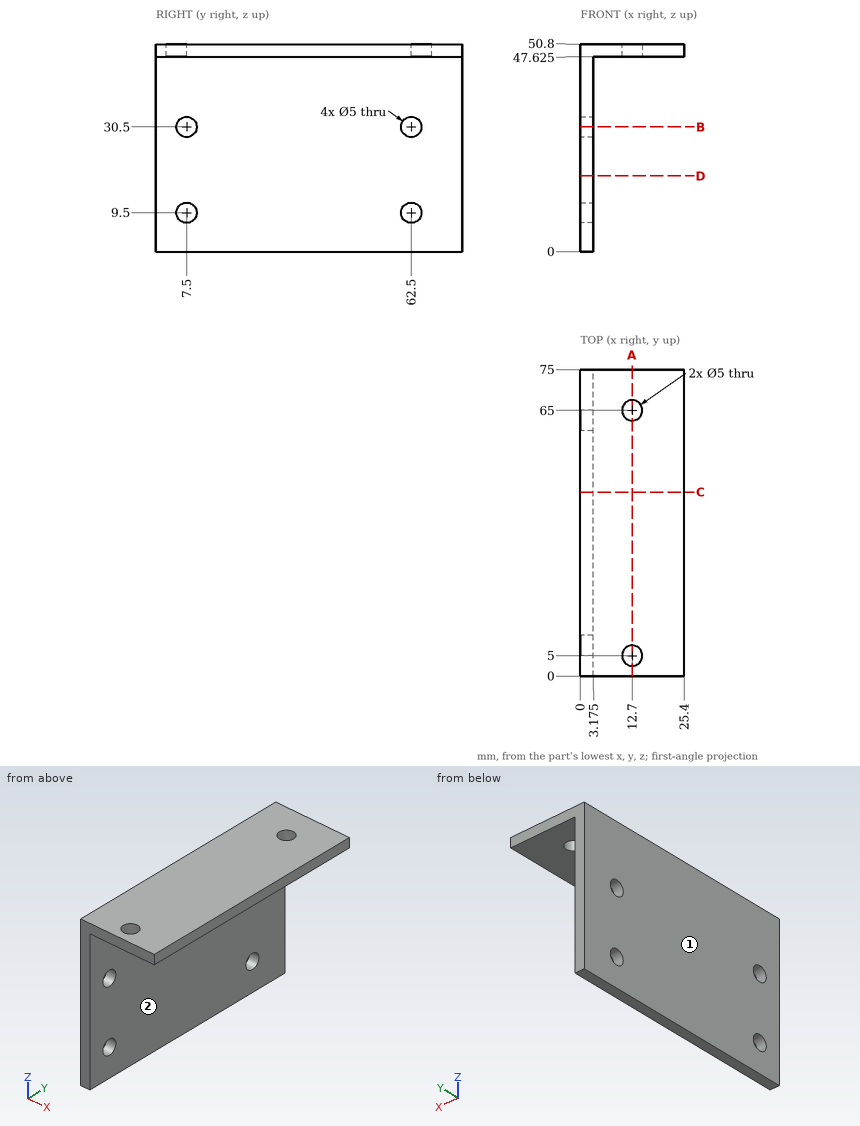
Can you work these out from the drawing? Everything is in mm from the part's minimum corner. A direction names the side the tool comes from. Round coordinates to 2 decimals unless told otherwise and drop trailing zeros. Write each loop counter-clockwise with the first axis right and the second up, starting at its lowest first coordinate (ties: lowest second). Pieces come first, ordered by that corner, then holes. Notation, with made-up numbers: (75, -27.5) - (124, -27.5) arc R27 ccw to (124, -0.5) - close; hole circle Ø11 at (50, 48.25). An arc over 180 degrees is marked (long way). Use a Markdown table: item, result.
Q1. I want a section at A-A (x = 12.7). List the corners of the cut face in (y, z) for me (3 decimals), plus the area to 3 significant figures.
Output values:
| item | result |
|---|---|
| outline | (0, 47.625) - (2.5, 47.625) - (2.5, 50.8) - (0, 50.8) - close; (7.5, 47.625) - (62.5, 47.625) - (62.5, 50.8) - (7.5, 50.8) - close; (67.5, 47.625) - (75, 47.625) - (75, 50.8) - (67.5, 50.8) - close |
| area | 206 mm2 |
Q2. For pin 1 (6.5 mm diameter, centred on y = 7.5, z = 30.5, fed in from +X) (3 decimals); pin 2 (3 mm diameter, centred on y = 62.5, z = 9.5, fed in from -X); pin 3 (11 mm diameter, centred on x = 9.5, y = 22, fed in from -Z) (3 decimals), each with a flat end and sliding along its axis, tell me the tip position at first contact or that it passes through.
Output values:
| item | result |
|---|---|
| pin 1 | x = 3.175 |
| pin 2 | through |
| pin 3 | z = 47.625 |
Q3. I want a section at D-D (z = 18.5). List the corners of the cut face in (x, y) for me (3 decimals), plus the area to 3 significant figures.
Output values:
| item | result |
|---|---|
| outline | (0, 0) - (3.175, 0) - (3.175, 75) - (0, 75) - close |
| area | 238 mm2 |
Q4. Please list where these lines run through material, in increasing order: L1, parallel to Y at x = 2.15, z = 9.5; L2, parallel to Y at x = 12.7, z = 49.8; L3, parallel to X at y = 66.5, z = 8 (3 decimals).
Output values:
| item | result |
|---|---|
| L1 | 0 to 5, 10 to 60, 65 to 75 |
| L2 | 0 to 2.5, 7.5 to 62.5, 67.5 to 75 |
| L3 | 0 to 3.175 |
Q5. I want a section at B-B (z = 30.5). List the corners of the cut face in (x, y) for me (3 decimals), plus the area to 3 significant figures.
Output values:
| item | result |
|---|---|
| outline | (0, 0) - (3.175, 0) - (3.175, 5) - (0, 5) - close; (0, 10) - (3.175, 10) - (3.175, 60) - (0, 60) - close; (0, 65) - (3.175, 65) - (3.175, 75) - (0, 75) - close |
| area | 206 mm2 |
Q6. I want a section at C-C (y = 45). List the corners of the cut face in (x, z) for me (3 decimals), plus the area to 3 significant figures.
Output values:
| item | result |
|---|---|
| outline | (0, 0) - (3.175, 0) - (3.175, 47.625) - (25.4, 47.625) - (25.4, 50.8) - (0, 50.8) - close |
| area | 232 mm2 |
Q7. For the marked faces 1 and 2, which set-ups out of +Z, -Z, +X, -X, +Y, -Y let a thin tool reach every point of the face, with its end or its side?
Output values:
| item | result |
|---|---|
| face 1 | +Z, -Z, -X, +Y, -Y |
| face 2 | -Z, +X, +Y, -Y |
